Part model, mm, in its own coordinate system. A direction names the side the tool comes from. Give positions to 0.01 mm unless a question says otherwise; leave off trailing zeros. Write each loop counter-clockwise with the first axis right and the second up, starting at its lowest first coordinate (ties: lowest second). Pieces come first, ordered by that corner, then holes.
from build123d import *

# Parameters (mm, degrees)
F0_R            = 37.5
F1_DEPTH        = 10
F2_R            = 37.5
F2_R_2          = 14
F3_DEPTH        = 4
F5_D            = 5
F5_CBORE_D      = 10
F5_CBORE_DEPTH  = 5
F5_COPIES_COUNT = 4
F7_D            = 4.1
F7_COPIES_COUNT = 4


# Not quite as in the source:
# - a pattern or mirror of a feature is missing from the dataset's text; its kind, count and spacing are read off the source's solid
# - a feature names something its author has since deleted; it is built from what else it names


with BuildPart() as f1:
    # F0 (on Top) → F1 (new body)
    with BuildSketch(Plane.XY):
        Circle(F0_R)
    extrude(amount=F1_DEPTH)

    # F2 (on face) → F3 (cut)
    with BuildSketch(Plane.XY.offset(10)):
        Circle(F2_R)
        Circle(F2_R_2, mode=Mode.SUBTRACT)
    extrude(amount=-F3_DEPTH, mode=Mode.SUBTRACT)

    # F5 (through all)
    with Locations(Plane.XY.offset(6)):
        with Locations((0, 28)):
            f5 = CounterBoreHole(F5_D / 2, F5_CBORE_D / 2, F5_CBORE_DEPTH)

    # F5_copies: F5 ×4 about axis
    f5_copies_axis = Axis((0, 0, 0), (0, 0, 1))
    for i in range(1, F5_COPIES_COUNT):
        add(f5.rotate(f5_copies_axis, i * 360 / F5_COPIES_COUNT), mode=Mode.SUBTRACT)

    # F7 (through all)
    with Locations(Plane(origin=(0, 0, 0), x_dir=(1, 0, 0), z_dir=(0, 0, -1))):
        with Locations((-12.0208152802, 12.0208152802)):
            f7 = Hole(F7_D / 2)

    # F7_copies: F7 ×4 about axis
    f7_copies_axis = Axis((0, 0, 0), (0, 0, 1))
    for i in range(1, F7_COPIES_COUNT):
        add(f7.rotate(f7_copies_axis, i * 360 / F7_COPIES_COUNT), mode=Mode.SUBTRACT)


solid = f1.part
1) Drill centre lines: L1, parallel to Z at x = 20, y = 29.5; L2, parallel to X at y = -30, z = 2.5; L3, parallel to X at y = -12.5, z = 5. Where is each one in solid material? Low to high.
Check result:
L1: z = 0 to 6
L2: x = -22.5 to -4.58, 4.58 to 22.5
L3: x = -35.36 to -14.01, -10.03 to 10.03, 14.01 to 35.36
2) 3-axis set-ups, long thin cutter, end or side, ignore diameter. For faces 1 (the cylindrical face through (-1.08, 23.12, 3.54)), 2 (the flat face through (0, 0, 10)): which of +Z, -Z, +X, -X, +Y, -Y reach the whole face in a straight line?
Check result:
face 1: +Z
face 2: +Z, +X, -X, +Y, -Y
3) Mould opens along X. For faces 3 (the cylindrical face through (-4.88, 37.18, 2.96)), 4 (the flat face through (-1, -16, 6)), 5 (the cylindrical face through (0.33, 30.48, 0.49)) say: +X half, -X half, draft (parallel to the pull), parting line (faces both ways), or undercut.
Check result:
face 3: parting line
face 4: draft
face 5: undercut
4) Saw through at C-C (z = 4.75). State how many separate pieces and enclosed holes the cut face has, and give its area (3 significant figures).
Check result:
separate pieces: 1
enclosed holes: 8
area: 4,050 mm2
5) Flat gauge pins, fed straight in: P1, Ø4, axis at x = 9, z = 5, coming from the -Y side; P2, Ø4, axis at x = -28, y = 0, coming from the +Z side; P3, Ø16, axis at x = 0, y = -28, coming from the +Z side; P4, Ø2, axis at x = 12.5, z = 8, coming from the -Y side. Where does each tip first touch, or does it go through?
Check result:
P1: stops at y = -36.84
P2: passes through
P3: stops at z = 6
P4: stops at y = -7.98
6) Saw through at A-A (x = 0). Write the cut outline in (y, z).
Check result:
outline: (-37.5, 0) - (-30.5, 0) - (-30.5, 1) - (-33, 1) - (-33, 6) - (-37.5, 6) - close; (-25.5, 0) - (25.5, 0) - (25.5, 1) - (23, 1) - (23, 6) - (14, 6) - (14, 10) - (-14, 10) - (-14, 6) - (-23, 6) - (-23, 1) - (-25.5, 1) - close; (30.5, 0) - (37.5, 0) - (37.5, 6) - (33, 6) - (33, 1) - (30.5, 1) - close
7) Saw through at D-D (x = -28). Write the cut outline in (y, z).
Check result:
outline: (-24.94, 0) - (-2.5, 0) - (-2.5, 1) - (-5, 1) - (-5, 6) - (-24.94, 6) - close; (2.5, 0) - (24.94, 0) - (24.94, 6) - (5, 6) - (5, 1) - (2.5, 1) - close
